Autodesk Inventor part; units mm, degrees
ref_plane "작업 평면1" through (-21.25, -9.325, 0) normal (0, -1, 0) x (1, 0, 0)
ref_plane "YZ Plane" through (0, 0, 0) normal (1, 0, 0) x (0, 1, 0)
ref_plane "XZ Plane" through (0, 0, 0) normal (0, 1, 0) x (-1, 0, 0)
sketch "스케치1" plane through (0, 0, 0) normal (0, 0, 1) x (1, 0, 0)
  line L0 (-21.25, 18.125) -> (21.25, 18.125)
  line L1 (21.25, 18.125) -> (21.25, -18.125)
  line L2 (21.25, -18.125) -> (-21.25, -18.125)
  line L3 (-21.25, -18.125) -> (-21.25, 18.125)
  line L4 (-21.25, 18.125) -> (21.25, -18.125) construction
  line L5 (21.25, 18.125) -> (-21.25, -18.125) construction
  point P0 (0, 0)
  dimension "d0" = 42.5
  dimension "d1" = 36.25
extrude "돌출1" add sketch "스케치1" along normal blind 3
fillet "모깎기1" radius 5 2 edges at (21.25, 18.125, 1.5) (-21.25, 18.125, 1.5)
ref_plane "작업 평면1" through (-21.25, -9.325, 0) normal (0, -1, 0) x (1, 0, 0)
sketch "스케치2" plane through (-21.25, -9.325, 0) normal (0, -1, 0) x (1, 0, 0)
  line L0 (21.25, 0) -> (21.25, -4)
  circle A0 centre (21.25, -4) radius 2
  circle A1 centre (21.25, -4) radius 4
  line L1 (21.25, 0) -> (26.25, 0)
  line L2 (0, 0) -> (42.5, 0) construction
  line L3 (26.25, 0) -> (25.1524, -4.878)
  line L4 (21.25, 0) -> (16.25, 0)
  line L5 (16.25, 0) -> (17.4292, -5.184)
  dimension "d6" = 4
  dimension "d7" = 4
  dimension "d8" = 8
  dimension "d9" = 10
extrude "돌출2" add sketch "스케치2" along normal blind 2 contours L1 L3 A1 | A1 L5 | A1 L5 L4 picked at (20.9261, -0.7066)
pattern_linear "직사각형 패턴1" count 2 spacing 22.5 along (0, 1, 0) of "돌출2"
sketch "스케치3" plane through (0, 0, 0) normal (0, 0, -1) x (-1, 0, 0)
  circle A0 centre (16.825, -2.325) radius 4.425
  line L0 (21.25, -18.125) -> (-21.25, -18.125)
  line L1 (0, 0) -> (0, 4.3779)
  circle A1 centre (-16.825, -2.325) radius 4.425
  line L2 (21.25, 13.125) -> (21.25, -18.125)
  line L3 (-19.075, -0.075) -> (-14.575, -0.075)
  line L4 (-14.575, -0.075) -> (-14.575, -4.575)
  line L5 (-14.575, -4.575) -> (-19.075, -4.575)
  line L6 (-19.075, -4.575) -> (-19.075, -0.075)
  line L7 (-19.075, -0.075) -> (-14.575, -4.575) construction
  line L8 (-14.575, -0.075) -> (-19.075, -4.575) construction
  line L9 (14.575, -4.575) -> (19.075, -4.575)
  line L10 (19.075, -4.575) -> (19.075, -0.075)
  line L11 (19.075, -0.075) -> (14.575, -0.075)
  line L12 (14.575, -0.075) -> (14.575, -4.575)
  line L13 (14.575, -4.575) -> (19.075, -0.075) construction
  line L14 (19.075, -4.575) -> (14.575, -0.075) construction
  dimension "d16" = 15.8
  dimension "d17" = 33.65
  dimension "d18" = 4.5
  dimension "d19" = 4.5
  dimension "d20" = 4.5
  dimension "d21" = 4.5
extrude "돌출3" add sketch "스케치3" along normal blind 2
sketch "스케치4" plane through (0, 0, 3) normal (0, 0, 1) x (1, 0, 0)
  line L0 (-21.25, -18.125) -> (21.25, -18.125)
  line L1 (21.25, -18.125) -> (21.25, 13.125)
  line L2 (-21.25, 13.125) -> (-21.25, -18.125)
  line L3 (-21.25, -17.825) -> (21.25, -17.825)
  point P0 (0, 0)
  dimension "d24" = 0.3
extrude "돌출4" cut sketch "스케치4" against normal blind 3
sketch "스케치5" plane through (0, 0, 3) normal (0, 0, 1) x (1, 0, 0)
  line L0 (15, 7) -> (17, 7)
  line L1 (17, 7) -> (17, -13)
  line L2 (17, -13) -> (15, -13)
  line L3 (15, -13) -> (15, 7)
  line L4 (15, 7) -> (17, -13) construction
  line L5 (17, 7) -> (15, -13) construction
  point P0 (0, 0)
  point P1 (16, -3)
  dimension "d27" = 2
  dimension "d28" = 20
  dimension "d32" = 3
  dimension "d33" = 16
extrude "돌출5" cut sketch "스케치5" against normal blind 0.5
chamfer "모따기1" distance 0.5 angle 45 4 edges at (15, -3, 3) (16, 7, 3) (17, -3, 3) (16, -13, 3)
sketch "스케치6" plane through (0, 0, 0) normal (0, 0, -1) x (-1, 0, 0)
  line L0 (-19.075, -0.075) -> (-19.075, -4.575)
  line L1 (-19.075, -4.575) -> (-14.575, -4.575)
  line L2 (-14.575, -4.575) -> (-14.575, -0.075)
  line L3 (-14.575, -0.075) -> (-19.075, -0.075)
  line L4 (14.575, -4.575) -> (19.075, -4.575)
  line L5 (19.075, -4.575) -> (19.075, -0.075)
  line L6 (19.075, -0.075) -> (14.575, -0.075)
  line L7 (14.575, -0.075) -> (14.575, -4.575)
  point P0 (0, 0)
extrude "돌출6" add sketch "스케치6" along normal blind 0.7
sketch "스케치9" plane through (-21.25, -9.325, 0) normal (0, 1, 0) x (1, 0, 0)
  arc A0 (25.1524, 4.878) -> (17.4292, 5.184) centre (21.25, 4) ccw
  line L0 (25.1524, 4.878) -> (17.3596, 4.878)
  line L1 (17.3596, 4.878) -> (17.3596, 8)
  line L2 (17.3596, 8) -> (25.1524, 8)
  line L3 (25.1524, 8) -> (25.1524, 4.878)
  line L4 (16.25, 0) -> (17.4292, 5.184)
  point P0 (21.25, 0)
  point P1 (21.25, 8)
extrude "돌출9" add sketch "스케치9" against normal blind 2 contours A0 L2 L3 | A0 L4 L1 L2
chamfer "모따기3" distance 1 angle 45 2 edges at (3.9024, -10.325, -8) (-3.8904, -10.325, -8)
pattern_linear "직사각형 패턴2" count 2 spacing 22.5 along (0, 1, 0) of "돌출9", "모따기3"
properties part number "버튼 스위치 상단"
Can you work these out from the model? Positions are in its coordinate system, mm. A direction names the side the tool comes from. Coordinates: 2 decimals unless noted, no trailing zeros. Loops run counter-clockwise (first coordinate to the right, second up) from the corner with the lowest first, then second, coordinate; pieces in that order, holes last.
1) Imagine slicing it at B-B on z = -4. List the corners of the cut face in (x, y) for me (3 decimals), plus the area to 3 significant figures.
2) Imagine slicing it at D-D on x = 10. List the corners of the cut face in (y, z) for me (3 decimals), plus the area to 3 significant figures.
3) Imagine slicing it at A-A on x = 0. List the corners of the cut face in (y, z) for me (3 decimals).
4) For pin 1 (1.6 mm diameter, centred on y = 12, z = -6.5, fed in from +X); pin 2 (5 mm diameter, centred on x = 0, z = -4, fed in from -Y) (3 decimals); pin 3 (1 mm diameter, centred on x = 17.5, z = -1.5, fed in from -Y), each with a flat end and sliding along its axis, tell me the tip position at first contact or that it passes through.
5) Thinking about a two-plate mould opening in X: for faces 1 (the flat face through (14, -2, -2)), 2 (the cylindrical face through (-19.746, 16.699, 1.521)), 3 (the flat face through (0, 0, 0)), which applies, pulls with the +X half, pulls with the -X half, needs draft (parallel to the pull), parting line crosses it, or undercut?
6) Which directions (+Z, -Z, +X, -X, +Y, -Y) give clear straight access to the entire face, cutting with the end or side of a thin tool? Please do faces 4 (the flat face through (3.902, -10, -6)), 5 (the flat face through (1, -9.325, -2)), 6 (the flat face through (1, 13.175, -2)), 7 (the flat face through (17, -2, -0.7)), 8 (the flat face through (-3.89, 12, -6)).
7) I need wall thicknesses on probe 1 along Z at (x, y) = (0, -10); probe 2 along Y at (x, z) = (-2, -5.75) (3 decimals); probe 3 along Z at (x, y) = (4, 1). Which ranges of each line are inside material? Lowest first, please.
Completed:
1. outline: (-4.09, -11.325) - (-2, -11.325) - (-2, -9.325) - (-4.09, -9.325) - close; (-4.09, 11.175) - (-2, 11.175) - (-2, 13.175) - (-4.09, 13.175) - close; (2, -11.325) - (4.1, -11.325) - (4.1, -9.325) - (2, -9.325) - close; (2, 11.175) - (4.1, 11.175) - (4.1, 13.175) - (2, 13.175) - close
1. area: 16.8 mm2
2. outline: (-17.825, 0) - (18.125, 0) - (18.125, 3) - (-17.825, 3) - close
2. area: 108 mm2
3. outline: (-17.825, 0) - (-11.325, 0) - (-11.325, -2) - (-9.325, -2) - (-9.325, 0) - (11.175, 0) - (11.175, -2) - (13.175, -2) - (13.175, 0) - (18.125, 0) - (18.125, 3) - (-17.825, 3) - close; (-11.325, -8) - (-9.325, -8) - (-9.325, -6) - (-11.325, -6) - close; (11.175, -8) - (13.175, -8) - (13.175, -6) - (11.175, -6) - close
4. pin 1: stops at x = 3.9
4. pin 2: stops at y = -11.325
4. pin 3: stops at y = -6.75
5. face 1: needs draft
5. face 2: pulls with the -X half
5. face 3: undercut
6. face 4: -Z, +X, +Y, -Y
6. face 5: -Z, +X, -X
6. face 6: -Z, +X, -X, +Y
6. face 7: -Z
6. face 8: -Z, -X, +Y, -Y
7. probe 1: z = -8 to -6, -2 to 3
7. probe 2: y = -11.325 to -9.325, 11.175 to 13.175
7. probe 3: z = 0 to 3
